from build123d import *

# Parameters (mm, degrees)
F0_W     = 38.1
F0_H     = 57.15
F1_DEPTH = 101.6
F2_R     = 5.15112
F3_DEPTH = 19.05


with BuildPart() as f1:
    # F0 (on Front) → F1 (new body)
    with BuildSketch(Plane.XZ):
        with Locations((19.05, 28.575)):
            Rectangle(F0_W, F0_H)
    extrude(amount=F1_DEPTH)

    # F2 (on face) → F3 (cut)
    with BuildSketch(Plane.XY.offset(57.15)):
        with Locations((19.05, -25.4)):
            Circle(F2_R)
        with Locations((19.05, -76.2)):
            Circle(F2_R)
    extrude(amount=-F3_DEPTH, mode=Mode.SUBTRACT)


solid = f1.part
The listing builds one solid part. Answer for the finished solid, in the listing's coordinates (mm). A direction names the side the tool comes from. Give positions to 0.01 mm unless a question says otherwise; leave off trailing zeros. Write each loop counter-clockwise with the first axis right and the second up, starting at its lowest first coordinate (ties: lowest second). Pieces come first, ordered by that corner, then holes. Notation, with made-up numbers: (79, 84) -> (122, 84) arc R19 ccw to (122, 101) -> close; hole circle Ø9 at (-17, 2.25). An arc over 180 degrees is marked (long way). One line per question, with ' | ' between items. Start each with the question number.
1. Find the intervals of material crossed by probe 1 along Y at (x, z) = (19.05, 51.5); probe 2 along X at (y, z) = (-76, 46); probe 3 along X at (y, z) = (-23, 45), in increasing order.
2. For a pull along Y with two mould halves and no side action, classify faces 1 (the flat face through (19, 0, 29)), 2 (the cylindrical face through (15.25, -21.92, 47.76)), 3 (the flat face through (19, -101.6, 29)) as pulls with the +Y half, pulls with the -Y half, needs draft (parallel to the pull), parting line crosses it, or undercut.
3. Section A-A (y = -25.4) is taken. Determine the outline of the cut face in (x, z), plus the area to 3 significant figures.
4. For faces 4 (the flat face through (19, -50, 0)), 5 (the cylindrical face through (15.25, -72.72, 47.76)), determine the directions among +Z, -Z, +X, -X, +Y, -Y from which every point of the face is accessible in a straight line to the end or side of a thin tool.
5. Section B-B (x = 19.05) is taken. Determine the outline of the cut face in (y, z), plus the area to 3 significant figures.
Response values:
1) probe 1: -101.6 to -81.35, -71.05 to -30.55, -20.25 to 0 | probe 2: 0 to 13.9, 24.2 to 38.1 | probe 3: 0 to 14.49, 23.61 to 38.1
2) face 1: pulls with the +Y half | face 2: undercut | face 3: pulls with the -Y half
3) outline: (0, 0) -> (38.1, 0) -> (38.1, 57.15) -> (24.2, 57.15) -> (24.2, 38.1) -> (13.9, 38.1) -> (13.9, 57.15) -> (0, 57.15) -> close | area: 1,980 mm2
4) face 4: -Z, +X, -X, +Y, -Y | face 5: +Z
5) outline: (-101.6, 0) -> (0, 0) -> (0, 57.15) -> (-20.25, 57.15) -> (-20.25, 38.1) -> (-30.55, 38.1) -> (-30.55, 57.15) -> (-71.05, 57.15) -> (-71.05, 38.1) -> (-81.35, 38.1) -> (-81.35, 57.15) -> (-101.6, 57.15) -> close | area: 5,410 mm2
